Read the model definition and answer for the solid it produces. Units are mm, in the model's axes. Face numbers are marked on the shaded views. A direction names the side the tool comes from. Coordinates: 2 decimals unless noted, no trailing zeros. Order: outer loops, then holes, each group sorted by start corner. A loop starts at its lowest first (then second) coordinate and runs counter-clockwise, first axis right, second up. Notation, with made-up numbers: M -30.5,-36 L 20.5,-36 A17 ccw 20.5,-23 Z; hole C 47,11.25 d9. An arc over 180 degrees is marked long. Put each result on its own line as item: value.
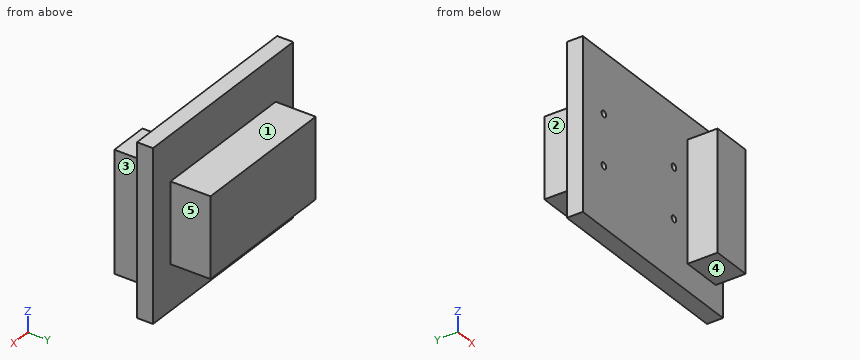
from build123d import *

# Parameters (mm, degrees)
SKETCH_1_W          = 100
SKETCH_1_H          = 85
EXTRUDE_1_DEPTH     = 8
SKETCH_2_W          = 75
SKETCH_2_H          = 40
EXTRUDE_2_DEPTH     = 20
SKETCH_3_W          = 20
SKETCH_3_H          = 60
EXTRUDE_3_DEPTH     = 15
SKETCH_4_R          = 1.6
CUT_EXTRUDE_1_DEPTH = 8


with BuildPart() as part:
    # 草图1 → 凸台-拉伸1 (new body)
    with BuildSketch(Plane(origin=(0, 0, 0), x_dir=(1, 0, 0), z_dir=(0, 1, 0))):
        Rectangle(SKETCH_1_W, SKETCH_1_H)
    extrude(amount=EXTRUDE_1_DEPTH)

    # 草图2 → 凸台-拉伸2 (add)
    with BuildSketch(Plane(origin=(0, 8, 0), x_dir=(1, 0, 0), z_dir=(0, 1, 0))):
        Rectangle(SKETCH_2_W, SKETCH_2_H)
    extrude(amount=EXTRUDE_2_DEPTH)

    # 草图3 → 凸台-拉伸3 (add)
    with BuildSketch(Plane.XZ):
        with Locations((34.768700032, 0.777091897)):
            Rectangle(SKETCH_3_W, SKETCH_3_H)
    extrude(amount=EXTRUDE_3_DEPTH)

    # 草图4 → 切除-拉伸1 (cut)
    with BuildSketch(Plane.XZ):
        with Locations((15, -12.5)):
            Circle(SKETCH_4_R)
        with Locations((15, 12.5)):
            Circle(SKETCH_4_R)
        with Locations((-35, 12.5)):
            Circle(SKETCH_4_R)
        with Locations((-35, -12.5)):
            Circle(SKETCH_4_R)
    extrude(amount=-CUT_EXTRUDE_1_DEPTH, mode=Mode.SUBTRACT)


solid = part.part
Q1. Given pin 1 (6 mm diameter, centred on y = 15, z = 0.5, fed in from -X); pin 2 (3 mm diameter, centred on x = 15, z = 12.5, fed in from -Y); pin 3 (4 mm diameter, centred on x = -30.5, z = 27.5, fed in from +Y); pin 4 (2 mm diameter, centred on x = -29.5, y = -2.5, fed in from +Z), each flat-ended and moving along its own axis, determine where each tip first touches the part or whether it passes through.
Answers below:
pin 1: stops at x = -37.5
pin 2: stops at y = 8
pin 3: stops at y = 8
pin 4: passes through
Q2. Consider line 1 along Z through (x, y) = (15, 5); line 2 along X through (y, z) = (5, 12); line 3 along Z through (x, y) = (12.5, 24). Determine where each line is inside the solid, lowest interval first.
Answers below:
line 1: z = -42.5 to -14.1, -10.9 to 10.9, 14.1 to 42.5
line 2: x = -50 to -36.52, -33.48 to 13.48, 16.52 to 50
line 3: z = -20 to 20
Q3. Find section D-D on y = 11. Write down the section's boundary in (x, z), plus the area to 3 significant figures.
Answers below:
outline: M -37.5,-20 L 37.5,-20 L 37.5,20 L -37.5,20 Z
area: 3,000 mm^2
Q4. A tool of negligible diameter and unlimited length cuts with its end or side. For the marked faces 1, 2, 3, 4 and 5, from which of +Z, -Z, +X, -X, +Y, -Y can it reach the whole face along a straight path? Write none if from no direction.
Answers below:
face 1: +Z, +X, -X, +Y
face 2: +Z, -Z, -X, +Y
face 3: +Z, -Z, +X, -Y
face 4: -Z, +X, -X, -Y
face 5: +Z, -Z, +X, +Y
Q5. Find section A-A on z = 28.5. Write down the section's boundary in (x, y), plus the area to 3 significant figures.
Answers below:
outline: M -50,0 L 24.77,0 L 24.77,-15 L 44.77,-15 L 44.77,0 L 50,0 L 50,8 L -50,8 Z
area: 1,100 mm^2
Q6. Find section B-B on x = 15. Write down the section's boundary in (y, z), plus the area to 3 significant figures.
Answers below:
outline: M 0,-42.5 L 8,-42.5 L 8,-20 L 28,-20 L 28,20 L 8,20 L 8,42.5 L 0,42.5 L 0,14.1 L 8,14.1 L 8,10.9 L 0,10.9 L 0,-10.9 L 8,-10.9 L 8,-14.1 L 0,-14.1 Z
area: 1,430 mm^2
Q7. Find section C-C on z = -12.5. Write down the section's boundary in (x, y), plus the area to 3 significant figures.
Answers below:
outline: M -50,0 L -36.6,0 L -36.6,8 L -33.4,8 L -33.4,0 L 13.4,0 L 13.4,8 L 16.6,8 L 16.6,0 L 24.77,0 L 24.77,-15 L 44.77,-15 L 44.77,0 L 50,0 L 50,8 L 37.5,8 L 37.5,28 L -37.5,28 L -37.5,8 L -50,8 Z
area: 2,550 mm^2
